Geometry: final body of the model. Coordinates: model frame, mm. A direction names the side the tool comes from. Coordinates: 2 decimals unless noted, no trailing zeros. Write each loop counter-clockwise with the first axis right and the second up, starting at its lowest first coordinate (ties: lowest second). Pieces come first, ordered by that corner, then holes.
from build123d import *

# Parameters (mm, degrees)
SKETCH1_R           = 12.288018633
SKETCH1_R_2         = 13.402342443
SKETCH1_R_3         = 5.966655134
BOSS_EXTRUDE1_DEPTH = 10


with BuildPart() as part:
    # Sketch1 → Boss-Extrude1 (new body)
    with BuildSketch(Plane.XY):
        with BuildLine():
            Line((-43.16670826, -100.459006624), (-43.16670826, -144.386357681))
            Line((-43.16670826, -144.386357681), (-43.16670826, -202.977586365))
            Line((-43.16670826, -202.977586365), (-19.89608029, -202.977586365))
            Line((-19.89608029, -202.977586365), (-19.89608029, -144.386357681))
            Line((-19.89608029, -144.386357681), (20.715262102, -144.386357681))
            Line((20.715262102, -144.386357681), (20.715262102, -202.977586365))
            Line((20.715262102, -202.977586365), (41.349988273, -202.977586365))
            Line((41.349988273, -202.977586365), (41.349988273, -144.386357681))
            Line((41.349988273, -144.386357681), (41.349988273, -100.459006624))
            Line((41.349988273, -100.459006624), (85.500022586, -100.459006624))
            Line((85.500022586, -100.459006624), (85.500022586, -144.386357681))
            Line((85.500022586, -144.386357681), (98.553668355, -144.386357681))
            Line((98.553668355, -144.386357681), (98.553668355, -100.459006624))
            Line((98.553668355, -100.459006624), (98.553668355, -85.011306082))
            Line((98.553668355, -85.011306082), (41.349988273, -85.011306082))
            Line((41.349988273, -85.011306082), (41.349988273, -57.873752711))
            ThreePointArc((41.349988273, -57.873752711), (1.129346742, 71.119036544), (-43.16670826, -56.531655566))
            Line((-43.16670826, -56.531655566), (-43.16670826, -85.011306082))
            Line((-43.16670826, -85.011306082), (-98.217954904, -85.011306082))
            Line((-98.217954904, -85.011306082), (-98.217954904, -100.459006624))
            Line((-98.217954904, -100.459006624), (-98.217954904, -143.510977861))
            Line((-98.217954904, -143.510977861), (-80.329625517, -143.510977861))
            Line((-80.329625517, -143.510977861), (-80.329625517, -100.459006624))
            Line((-80.329625517, -100.459006624), (-43.16670826, -100.459006624))
        make_face()
        with Locations((-33.517420804, 16.851364033)):
            Circle(SKETCH1_R, mode=Mode.SUBTRACT)
        with Locations((30.688490145, 16.851364033)):
            Circle(SKETCH1_R_2, mode=Mode.SUBTRACT)
        with Locations((0, -13.237752907)):
            Circle(SKETCH1_R_3, mode=Mode.SUBTRACT)
    extrude(amount=BOSS_EXTRUDE1_DEPTH)


solid = part.part
Item 1: Section A-A, the plane y = -106. Output: boundary loops of the cut face in (x, z).
Derived:
outline: (-98.22, 0) - (-80.33, 0) - (-80.33, 10) - (-98.22, 10) - close; (-43.17, 0) - (41.35, 0) - (41.35, 10) - (-43.17, 10) - close; (85.5, 0) - (98.55, 0) - (98.55, 10) - (85.5, 10) - close
Item 2: Pin query (flat end, axial travel): pin 1 (22 mm diameter, centred on x = -33.52, y = 16.85, fed in from -Z); pin 2 (3 mm diameter, centred on x = 76.5, z = 2, fed in from -Y); pin 3 (19 mm diameter, centred on x = 0, y = -13.24, fed in from -Z); pin 4 (5 mm diameter, centred on x = 76, z = 5, fed in from +Y). Return the tip coordinate at first contact, or that it passes through.
Derived:
pin 1: passes through
pin 2: stops at y = -100.46
pin 3: stops at z = 0
pin 4: stops at y = -85.01
Item 3: Section D-D, the plane x = -40. Output: boundary loops of the cut face in (y, z).
Derived:
outline: (-202.98, 0) - (6.41, 0) - (6.41, 10) - (-202.98, 10) - close; (27.29, 0) - (58.81, 0) - (58.81, 10) - (27.29, 10) - close
Item 4: Section C-C, the plane z = 8. Output: boundary loops of the cut face in (x, y), plus the area to 3 significant figures.
Derived:
outline: (-98.22, -143.51) - (-80.33, -143.51) - (-80.33, -100.46) - (-43.17, -100.46) - (-43.17, -202.98) - (-19.9, -202.98) - (-19.9, -144.39) - (20.72, -144.39) - (20.72, -202.98) - (41.35, -202.98) - (41.35, -100.46) - (85.5, -100.46) - (85.5, -144.39) - (98.55, -144.39) - (98.55, -85.01) - (41.35, -85.01) - (41.35, -57.87) arc R71.13 ccw (long way) to (-43.17, -56.53) - (-43.17, -85.01) - (-98.22, -85.01) - close; hole circle Ø24.58 at (-33.52, 16.85); hole circle Ø11.93 at (0, -13.24); hole circle Ø26.8 at (30.69, 16.85)
area: 27,000 mm2
Item 5: Section B-B, the plane x = 0. Output: boundary loops of the cut face in (y, z).
Derived:
outline: (-144.39, 0) - (-19.2, 0) - (-19.2, 10) - (-144.39, 10) - close; (-7.27, 0) - (71.13, 0) - (71.13, 10) - (-7.27, 10) - close
Item 6: Pull-direction query (X, two-part tool) for faces 5 (the flat face through (63, -100.459, 5)), 6 (the cylindrical face through (3.623, 71.036, 4.93)), 7 (the flat face through (-70, -85.011, 5)); classes: released by +X, released by -X, zero draft, split by the parting line, or undercut.
Derived:
face 5: undercut
face 6: split by the parting line
face 7: zero draft
Item 7: Set-up query: faces 1 (the flat face through (41.35, -72, 5)), 2 (the flat face through (-89, -143.511, 5)), 3 (the flat face through (92, -144.386, 5)), 4 (the flat face through (-80.33, -122, 5)). Return all of +Z, -Z, +X, -X, +Y, -Y with unobstructed straight access to the full face (end or side cutting, diameter ignored); none if empty.
Derived:
face 1: +Z, -Z, +X
face 2: +Z, -Z, -X, -Y
face 3: +Z, -Z, +X, -Y
face 4: +Z, -Z, -Y
Item 8: Material intervals for probe 1 along X at (y, z) = (-142, 9); probe 2 along Y at (x, z) = (0, 5.75); probe 3 along X at (y, z) = (-162.5, 8.25), sorted ascending.
Derived:
probe 1: x = -98.22 to -80.33, -43.17 to 41.35, 85.5 to 98.55
probe 2: y = -144.39 to -19.2, -7.27 to 71.13
probe 3: x = -43.17 to -19.9, 20.72 to 41.35
